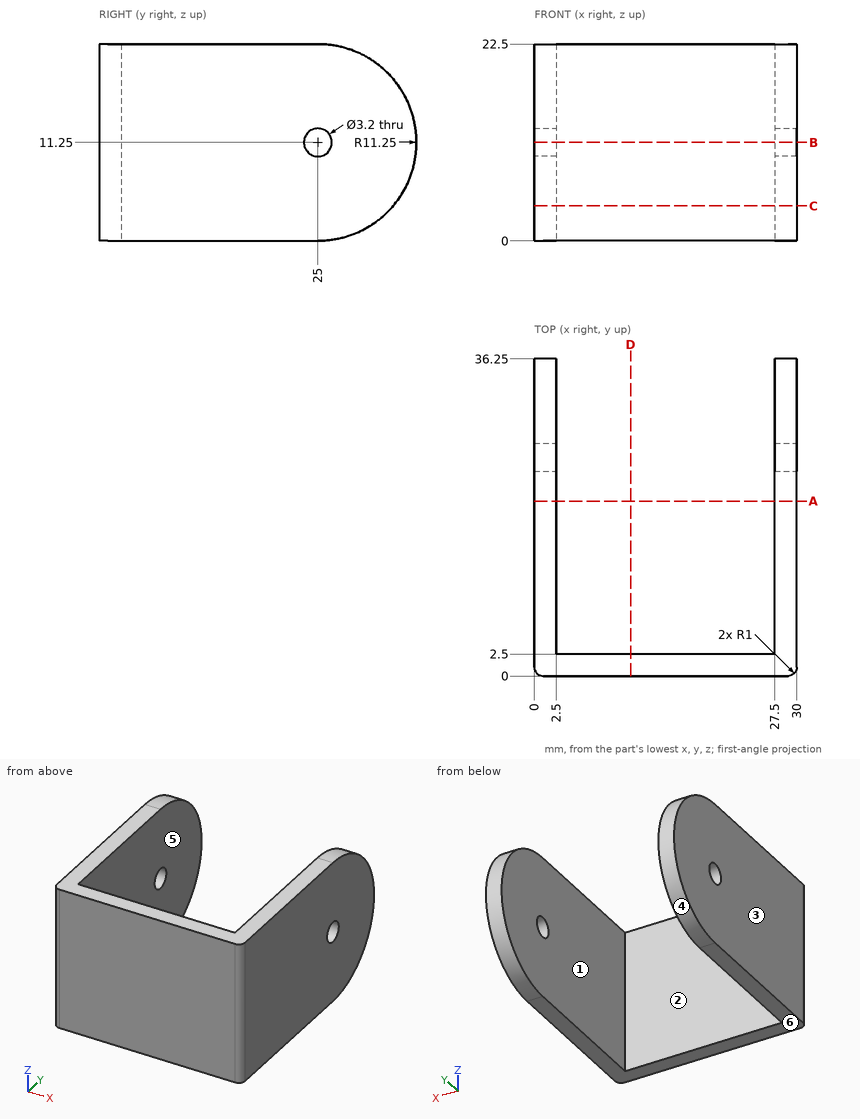
Verification items for this drawing (mm, ordinates from the low corner). A direction names the side the tool comes from. Give positions to 0.01 mm unless a question says otherwise; leave off trailing zeros. Loops run counter-clockwise (first coordinate to the right, second up) from the corner with the lowest first, then second, coordinate; pieces in that order, holes last.
1. Material ranges on probe 1 along X at (y, z) = (4, 7.75); probe 2 along Y at (x, z) = (1.8, 11.25); probe 3 along Y at (x, z) = (11, 6), recorded low to high.
Derived:
probe 1: x = 0 to 2.5, 27.5 to 30
probe 2: y = 0 to 23.4, 26.6 to 36.25
probe 3: y = 0 to 2.5
2. Tool access check on the marked faces 5 and 6. Record the directions out of +Z, -Z, +X, -X, +Y, -Y that give a thin tool (end or side, any length) a straight path to the whole face; none if there is none.
Derived:
face 5: +Z, -Z, +Y
face 6: -Z, +X, -X, +Y, -Y
3. Cross-section at B-B on z = 11.25. Record the cut outline in (x, y), and give its area (3 significant figures).
Derived:
outline: (0, 1) arc R1 ccw to (1, 0) - (29, 0) arc R1 ccw to (30, 1) - (30, 23.4) - (27.5, 23.4) - (27.5, 2.5) - (2.5, 2.5) - (2.5, 23.4) - (0, 23.4) - close; (0, 26.6) - (2.5, 26.6) - (2.5, 36.25) - (0, 36.25) - close; (27.5, 26.6) - (30, 26.6) - (30, 36.25) - (27.5, 36.25) - close
area: 227 mm2
4. Go/stop test with a flat-tipped pin: P1, Ø7, axis at x = 16.5, z = 11.5, coming from the +Y side. Record where the tip stops, or that it passes through.
Derived:
P1: stops at y = 2.5
5. Cross-section at D-D on x = 11. Record the cut outline in (y, z), and give its area (4 significant figures).
Derived:
outline: (0, 0) - (2.5, 0) - (2.5, 22.5) - (0, 22.5) - close
area: 56.25 mm2
6. Release check for a two-part mould opening along X. For the marked faces 1, 2, 3 and 4 record: +X half, -X half, draft (parallel to the pull), parting line (faces both ways), or undercut.
Derived:
face 1: undercut
face 2: undercut
face 3: -X half
face 4: draft
7. Cross-section at C-C on z = 4. Record the cut outline in (x, y).
Derived:
outline: (0, 1) arc R1 ccw to (1, 0) - (29, 0) arc R1 ccw to (30, 1) - (30, 33.6) - (27.5, 33.6) - (27.5, 2.5) - (2.5, 2.5) - (2.5, 33.6) - (0, 33.6) - close
8. Cross-section at A-A on y = 20. Record the cut outline in (x, z).
Derived:
outline: (0, 0) - (2.5, 0) - (2.5, 22.5) - (0, 22.5) - close; (27.5, 0) - (30, 0) - (30, 22.5) - (27.5, 22.5) - close
